The listing builds one solid part. Answer for the finished solid, in the listing's coordinates (mm). Face numbers are marked on the shaded views. A direction names the side the tool comes from. Coordinates: 2 decimals unless noted, no trailing zeros. Write each loop counter-clockwise with the first axis right and the second up, starting at its lowest first coordinate (ties: lowest second). Pieces come first, ordered by that corner, then holes.
Autodesk Inventor part; units mm, degrees
ref_plane "Work Plane1" through (4, 0, 0) normal (0, 0, 1) x (1, 0, 0)
ref_plane "YZ Plane" through (0, 0, 0) normal (1, 0, 0) x (0, 1, 0)
ref_plane "XZ Plane" through (0, 0, 0) normal (0, 1, 0) x (-1, 0, 0)
sketch "Sketch1" plane through (0, 0, 0) normal (0, 0, 1) x (1, 0, 0)
  line L0 (0, 0) -> (3.5, 0)
  line L1 (8, 1.7321) -> (8, 3)
  line L2 (8, 3) -> (0, 3)
  line L3 (8, 1.7321) -> (4.5, 1.7321)
  line L4 (4.5, 1.7321) -> (3.5, 0)
  line L5 (0, -0.6) -> (0, 3.6)
  line L6 (0, 3) -> (0, 0)
  dimension "d0" = 3.5
  dimension "d1" = 60
  dimension "d2" = 6
  dimension "d3" = 3.4641
  dimension "d5" = 8
revolve "Body" add sketch "Sketch1" angle 360 about axis through (0, 0, 0) along (1, 0, 0)
sketch "Sketch2" plane through (8, 0, 0) normal (1, 0, 0) x (0, 1, 0)
  circle A0 centre (0, 0) radius 1.7321
  line L0 (-0.866, 1.5) -> (0.866, 1.5)
  line L1 (0.866, 1.5) -> (1.7321, 0)
  line L2 (1.7321, 0) -> (0.866, -1.5)
  line L3 (0.866, -1.5) -> (-0.866, -1.5)
  line L4 (-0.866, -1.5) -> (-1.7321, 0)
  line L5 (-1.7321, 0) -> (-0.866, 1.5)
  point P0 (0, 0)
  point P1 (0, 0)
extrude "Slot" add sketch "Sketch2" against normal up to next contours L1 A0 | A0 L2 | L0 A0 | A0 L3 | L5 A0 | A0 L4
thread "Thread"
chamfer "Chamfer1" distance 0.6135 angle 45 1 edges at (8, -3, 0) measured on face at (5.3333, 2.9612, -0.4812)
chamfer "Chamfer2" distance 0.6135 angle 45 1 edges at (0, -3, 0) measured on face at (4.9244, 2.9612, -0.4812)
ref_plane "Work Plane1" through (4, 0, 0) normal (0, 0, 1) x (1, 0, 0)
equation "\"d8\" = NLG"
equation "\"d10\" = -0.5 * GD1 + 0.5 * NND"
equation "\"d11\" = FAWI"
equation "\"d34\" = -0.5 * GD1 + 0.5 * NND"
equation "\"d12\" = -0.5 * GD1 + 0.5 * NND"
equation "\"d13\" = FAWI"
equation "\"d35\" = -0.5 * GD1 + 0.5 * NND"
equation "\"d0\" = INTI"
equation "\"d2\" = NND"
equation "\"d3\" = 1.1547 * SW"
equation "\"d5\" = NLG"
equation "\"NND\" = 6"
equation "\"NLG\" = 8"
equation "\"INTI\" = 3.5"
equation "\"FAWI\" = 45deg"
equation "\"SW\" = 3"
equation "\"GD1\" = THREADDIA - 1.2269 * PTC"
equation "\"SPD\" = 4"
equation "\"GUL\" = 0.61345 * PTC"
equation "\"TOA\" = 30deg"
equation "\"THREADDIA\" = 6"
equation "\"PTC\" = 1"
equation "\"FAWI1\" = 45deg"
equation "\"GAL\" = 0.61345 * PTC"
equation "\"E0\" = 1.155 * SW"
properties part number "DIN 913 - M6 x 8" material "Steel, Mild"
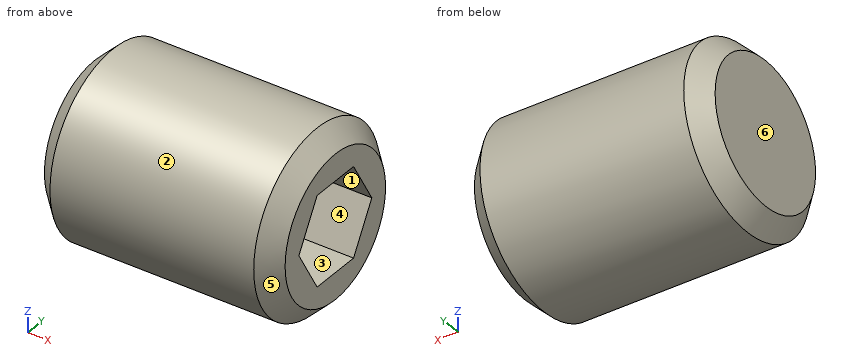
1. Section B-B on x = 6 is taken. Give the vertices of the cut face in (y, z).
Results found:
outline: circle Ø6 at (0, 0); hole (-1.73, 0) - (-0.87, -1.5) - (0.87, -1.5) - (1.73, 0) - (0.87, 1.5) - (-0.87, 1.5) - close
2. Find the intervals of material crossed by L1, parallel to Z at x = 5.25, y = 0.1; L2, parallel to Z at x = 6.5, y = -0.9; L3, parallel to Y at x = 4.5, z = 0.45, in increasing order.
Results found:
L1: z = -3 to -1.5, 1.5 to 3
L2: z = -2.86 to -1.44, 1.44 to 2.86
L3: y = -2.97 to -1.47, 1.47 to 2.97
3. A flat-ended cylindrical pin translates along its axis: P1, Ø1.5, axis at x = 2, y = -1.5, coming from the -Z side. Find the tip coordinate at first contact, or state that the pin passes through.
Results found:
P1: stops at z = -2.9
4. For a pull along Z with two mould halves and no side action, classify the marked faces 3, 4, 5 and 6 as pulls with the +Z half, pulls with the -Z half, needs draft (parallel to the pull), parting line crosses it, or undercut.
Results found:
face 3: undercut
face 4: undercut
face 5: parting line crosses it
face 6: needs draft
5. Section A-A on x = 2 is taken. Give the vertices of the cut face in (y, z), then the cut area to 3 significant figures.
Results found:
outline: circle Ø6 at (0, 0)
area: 28.3 mm2
6. A tool of negligible diameter and unlimited length cuts with its end or side. For the marked faces 1 and 2, from which of +Z, -Z, +X, -X, +Y, -Y can it reach the whole face along a straight path? Write none if from no direction.
Results found:
face 1: +X
face 2: +X, -X
